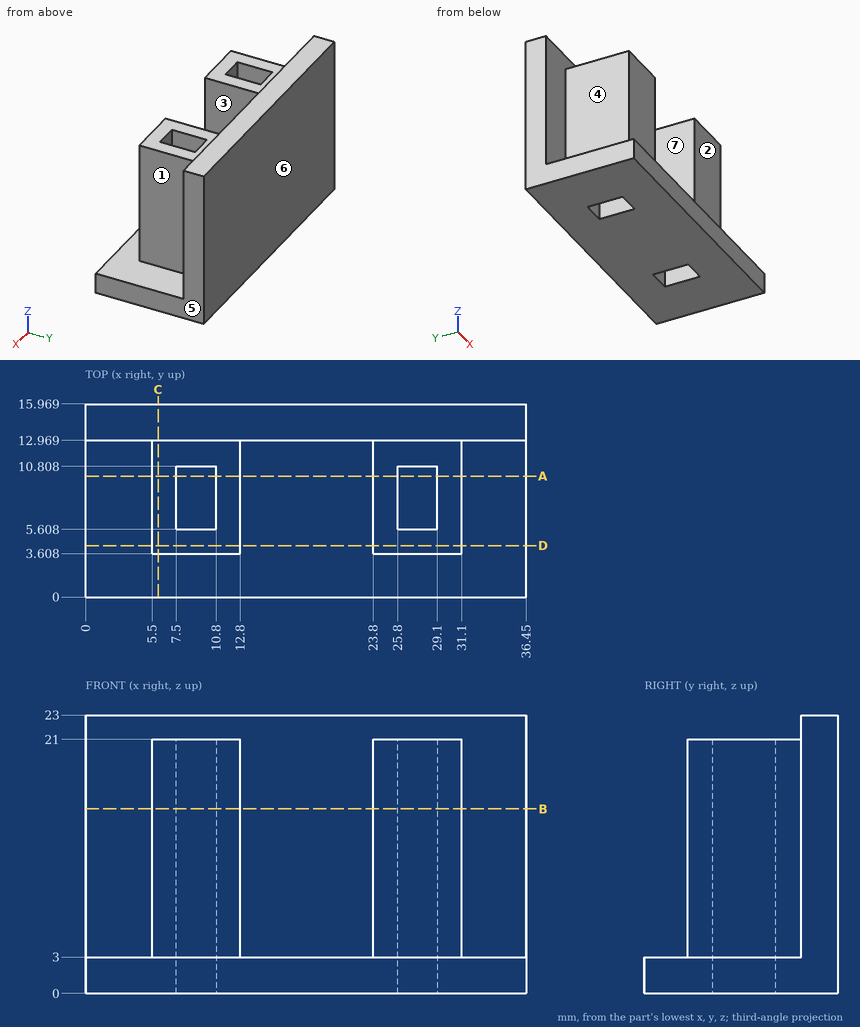
Could you check a few things on this drawing? It's one solid part, dimensions in mm from its lowest x, y, z. A direction names the side the tool comes from. Coordinates: 2 decimals unless noted, no trailing zeros. Order: outer loops, then holes, each group sorted by start corner. A loop starts at its lowest first (then second) coordinate and runs counter-clockwise, first axis right, second up.
1. I need wall thicknesses on line 1 (X direction, y = 8.75, z = 1.75); line 2 (X direction, y = 7.25, z = 4.5); line 3 (X direction, y = 4.75, z = 15). Which ranges of each line are inside material? Lowest first, please.
2. Thinking about a two-plate mould opening in X: for the marked faces 5, 6 and 7, which applies, +X half, -X half, draft (parallel to the pull), parting line (faces both ways), or undercut?
3. I'm going to push flat-ended pins straight in: pin 1 (1 mm diameter, centred on x = 28, z = 10, fed in from -Y); pin 2 (1.6 mm diameter, centred on y = 9, z = 15, fed in from -X); pin 3 (4 mm diameter, centred on x = 17, z = 8.5, fed in from -Y). Where does each tip first touch, or does it pass through?
4. If we section it at C-C (x = 6): Please give me the cut outline in (y, z), then the cut area to 3 significant figures.
5. For the marked faces 1, 2, 3 and 4, which set-ups out of +Z, -Z, +X, -X, +Y, -Y let a thin tool reach every point of the face, with its end or its side?
6. If we section it at B-B (z = 15.25): Please give me the cut outline in (x, y).
7. If we section it at A-A (y = 10): Please give me the cut outline in (x, z).
8. If we section it at D-D (y = 4.25): Please give me the cut outline in (x, z), then the cut area to 3 significant figures.
Entries:
1. line 1: x = 0 to 7.5, 10.8 to 25.8, 29.1 to 36.45
1. line 2: x = 5.5 to 7.5, 10.8 to 12.8, 23.8 to 25.8, 29.1 to 31.1
1. line 3: x = 5.5 to 12.8, 23.8 to 31.1
2. face 5: +X half
2. face 6: draft
2. face 7: undercut
3. pin 1: stops at y = 3.61
3. pin 2: stops at x = 5.5
3. pin 3: stops at y = 12.97
4. outline: (0, 0) - (15.97, 0) - (15.97, 23) - (12.97, 23) - (12.97, 21) - (3.61, 21) - (3.61, 3) - (0, 3) - close
4. area: 276 mm2
5. face 1: +Z, +X, -Y
5. face 2: +Z, +X, -X, -Y
5. face 3: +Z, -Y
5. face 4: +Z, -X, -Y
6. outline: (0, 12.97) - (5.5, 12.97) - (5.5, 3.61) - (12.8, 3.61) - (12.8, 12.97) - (23.8, 12.97) - (23.8, 3.61) - (31.1, 3.61) - (31.1, 12.97) - (36.45, 12.97) - (36.45, 15.97) - (0, 15.97) - close; hole (7.5, 5.61) - (10.8, 5.61) - (10.8, 10.81) - (7.5, 10.81) - close; hole (25.8, 5.61) - (29.1, 5.61) - (29.1, 10.81) - (25.8, 10.81) - close
7. outline: (0, 0) - (7.5, 0) - (7.5, 21) - (5.5, 21) - (5.5, 3) - (0, 3) - close; (10.8, 0) - (25.8, 0) - (25.8, 21) - (23.8, 21) - (23.8, 3) - (12.8, 3) - (12.8, 21) - (10.8, 21) - close; (29.1, 0) - (36.45, 0) - (36.45, 3) - (31.1, 3) - (31.1, 21) - (29.1, 21) - close
8. outline: (0, 0) - (36.45, 0) - (36.45, 3) - (31.1, 3) - (31.1, 21) - (23.8, 21) - (23.8, 3) - (12.8, 3) - (12.8, 21) - (5.5, 21) - (5.5, 3) - (0, 3) - close
8. area: 372 mm2
